Answer from the drawing. Dimensions are ordinates in mm from the lowest x, y and z of the part. Coordinates: 2 decimals unless noted, no trailing zeros. Order: outer loops, then holes, each group sorted by start corner. A loop starts at its lowest first (then second) coordinate and runs counter-clockwise, first axis right, second up. Notation, with made-up numbers: (9, 80) -> (18, 80) arc R21 cw to (18, 98) -> close; hole circle Ø5 at (-6.75, 37.5). An arc over 180 degrees is marked (long way). Answer in a Markdown table with one row per item.
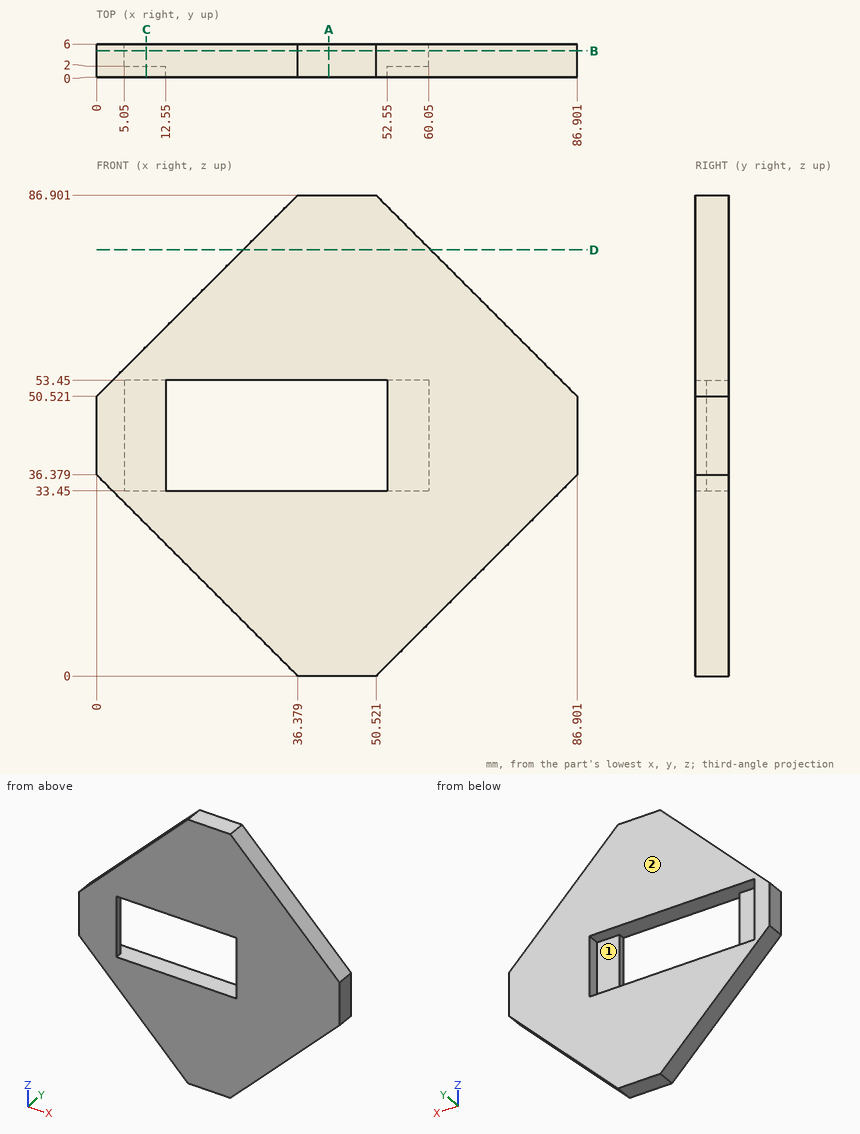
(1) A cutting plane is placed at B-B, the plane y = 4.75. Determine the outline of the cut face in (x, z).
Check values:
| item | result |
|---|---|
| outline | (0, 36.38) -> (36.38, 0) -> (50.52, 0) -> (86.9, 36.38) -> (86.9, 50.52) -> (50.52, 86.9) -> (36.38, 86.9) -> (0, 50.52) -> close; hole (5.05, 33.45) -> (60.05, 33.45) -> (60.05, 53.45) -> (5.05, 53.45) -> close |
(2) A cutting plane is placed at A-A, the plane x = 42. Determine the outline of the cut face in (y, z).
Check values:
| item | result |
|---|---|
| outline | (0, 0) -> (6, 0) -> (6, 33.45) -> (0, 33.45) -> close; (0, 53.45) -> (6, 53.45) -> (6, 86.9) -> (0, 86.9) -> close |
(3) For a pull along Z with two mould halves and no side action, classify the marked faces 1 and 2 as released by +Z, released by -Z, zero draft, split by the parting line, or undercut.
Check values:
| item | result |
|---|---|
| face 1 | undercut |
| face 2 | zero draft |
(4) Find the intervals of material crossed by line 1 along Z through (x, y) = (43, 2); line 2 along X through (y, z) = (2.8, 40); line 3 along Y through (x, z) = (11, 50), in increasing order. Write a range as from..to.
Check values:
| item | result |
|---|---|
| line 1 | 0..33.45, 53.45..86.9 |
| line 2 | 0..5.05, 60.05..86.9 |
| line 3 | 0..2 |
(5) A cutting plane is placed at C-C, the plane x = 9. Determine the outline of the cut face in (y, z), then the cut area to 3 significant figures.
Check values:
| item | result |
|---|---|
| outline | (0, 27.38) -> (6, 27.38) -> (6, 33.45) -> (2, 33.45) -> (2, 53.45) -> (6, 53.45) -> (6, 59.52) -> (0, 59.52) -> close |
| area | 113 mm² |
(6) A cutting plane is placed at D-D, the plane z = 77. Determine the outline of the cut face in (x, y), then the cut area to 3 significant figures.
Check values:
| item | result |
|---|---|
| outline | (26.48, 0) -> (60.42, 0) -> (60.42, 6) -> (26.48, 6) -> close |
| area | 204 mm² |
(7) Flat-ended cylindrical pins translate along their axes: pin 1 (4 mm diameter, centred on x = 56, z = 39.5, fed in from +Y); pin 2 (1.8 mm diameter, centred on x = 31.5, y = 3, fed in from +Z). Find the tip coordinate at first contact, or state that the pin passes through.
Check values:
| item | result |
|---|---|
| pin 1 | y = 2 |
| pin 2 | z = 82.92 |
